```python
from build123d import *

# Parameters (mm, degrees)
SKETCH1_W           = 82
SKETCH1_H           = 38
MAIN_DEPTH          = 3
SKETCH2_W           = 72.5
SKETCH2_H           = 25.5
LCD_CUTOUT_DEPTH    = 46.287967497
SKETCH3_W           = 41
SKETCH3_H           = 4.75
CONNECTOR_CUT_DEPTH = 1.5
SKETCH4_W           = 9.33307462
SKETCH4_H           = 11
CUT_EXTRUDE3_DEPTH  = 46.287967497
SKETCH6_W           = 82
SKETCH6_H           = 38
BOSS_EXTRUDE2_DEPTH = 2
SKETCH7_W           = 80.5
SKETCH7_H           = 36.5
CUT_EXTRUDE6_DEPTH  = 46.287967497
SKETCH8_W           = 41
SKETCH8_H           = 4.75
CUT_EXTRUDE7_DEPTH  = 46.323834789
SKETCH9_W           = 0.75
SKETCH9_H           = 11
BOSS_EXTRUDE3_DEPTH = 3
SKETCH10_W          = 38
SKETCH10_H          = 5
CUT_EXTRUDE8_DEPTH  = 1.2


with BuildPart() as part:
    # Sketch1 → main (new body)
    with BuildSketch(Plane(origin=(0, 0, 0), x_dir=(1, 0, 0), z_dir=(0, 1, 0))):
        Rectangle(SKETCH1_W, SKETCH1_H)
    extrude(amount=MAIN_DEPTH)

    # Sketch2 → LCD cutout (cut, through all)
    with BuildSketch(Plane(origin=(0, 3, 0), x_dir=(1, 0, 0), z_dir=(0, 1, 0))):
        Rectangle(SKETCH2_W, SKETCH2_H)
    extrude(amount=-LCD_CUTOUT_DEPTH, mode=Mode.SUBTRACT)

    # Sketch3 → connector cut (cut)
    with BuildSketch(Plane.XZ):
        with Locations((-14.5, -16.625)):
            Rectangle(SKETCH3_W, SKETCH3_H)
    extrude(amount=-CONNECTOR_CUT_DEPTH, mode=Mode.SUBTRACT)

    # Sketch4 → Cut-Extrude3 (cut, through all)
    with BuildSketch(Plane(origin=(0, 3, 0), x_dir=(1, 0, 0), z_dir=(0, 1, 0))):
        with Locations((36.888390736, 0)):
            Rectangle(SKETCH4_W, SKETCH4_H)
    extrude(amount=-CUT_EXTRUDE3_DEPTH, mode=Mode.SUBTRACT)

    # Sketch6 → Boss-Extrude2 (add)
    with BuildSketch(Plane(origin=(0, 0, 0), x_dir=(1, 0, 0), z_dir=(0, 1, 0))):
        Rectangle(SKETCH6_W, SKETCH6_H)
    extrude(amount=-BOSS_EXTRUDE2_DEPTH)

    # Sketch7 → Cut-Extrude6 (cut, through all)
    with BuildSketch(Plane(origin=(0, 0, 0), x_dir=(1, 0, 0), z_dir=(0, 1, 0))):
        Rectangle(SKETCH7_W, SKETCH7_H)
    extrude(amount=-CUT_EXTRUDE6_DEPTH, mode=Mode.SUBTRACT)

    # Sketch8 → Cut-Extrude7 (cut, through all)
    with BuildSketch(Plane.XZ.offset(-1.5)):
        with Locations((-14.5, -16.625)):
            Rectangle(SKETCH8_W, SKETCH8_H)
    extrude(amount=CUT_EXTRUDE7_DEPTH, mode=Mode.SUBTRACT)

    # Sketch9 → Boss-Extrude3 (add)
    with BuildSketch(Plane(origin=(0, 0, 0), x_dir=(1, 0, 0), z_dir=(0, 1, 0))):
        with Locations((40.625, 0)):
            Rectangle(SKETCH9_W, SKETCH9_H)
    extrude(amount=BOSS_EXTRUDE3_DEPTH)

    # Sketch10 → Cut-Extrude8 (cut)
    with BuildSketch(Plane.ZY.offset(41)):
        with Locations((0, 0.5)):
            Rectangle(SKETCH10_W, SKETCH10_H)
    extrude(amount=-CUT_EXTRUDE8_DEPTH, mode=Mode.SUBTRACT)


solid = part.part
```
Work out the finished part from the listing and answer in its coordinate system (mm). A direction names the side the tool comes from. Give positions to 0.01 mm unless a question says otherwise; leave off trailing zeros. Order: outer loops, then holes, each group sorted by start corner. A loop starts at its lowest first (then second) coordinate and runs counter-clockwise, first axis right, second up. Notation, with made-up numbers: (76.25, -26.75) - (125.25, -26.75) arc R29 ccw to (125.25, 9.25) - close; hole circle Ø1 at (28, 51.5). An arc over 180 degrees is marked (long way). One line per item, written item: value. Start each with the question number.
1. Consider line 1 (Z direction, x = -18, y = 1.4); line 2 (Z direction, x = 34, y = 1.05); line 3 (X direction, y = 0.7, z = 8.5). Determine where each line is inside the solid, lowest interval first.
2. Each of these flat-tipped pins is pushed along its axis until it touches: pin 1 Ø5 at (x, z) = (-19.5, -16.5) entering from -Y; pin 2 Ø0.6 at (x, y) = (-7, -1.5) entering from -Z; pin 3 Ø1.6 at (x, y) = (-6.5, 1) entering from -Z. Where does it stop, or does it pass through?
3. Section A-A, the plane z = -7 is taken. Write down the section's boundary in (x, y).
4. Section C-C, the plane y = -0.85 is taken. Write down the section's boundary in (x, z), then the cut area to 3 significant figures.
5. For a pull along Z with two mould halves and no side action, classify faces 5 (the face through (-15, 1.5, -17)), 6 (the face through (-15, 1, -14.25)), 7 (the face through (-37, -1, -18.25)), 8 (the face through (40.25, 0, 0)) as released by +Z, released by -Z, zero draft, split by the parting line, or undercut.
6. Section B-B, the plane x = 29 is taken. Write down the section's boundary in (y, z).
7. Which of the six approach directions +Z, -Z, +X, -X, +Y, -Y give full straight-line access (tool end or side, diameter ignored) to faces 1 (the face through (9, 1, -19)), 2 (the face through (0, -1, 18.25)), 3 (the face through (-1, 2, 12.75)), 4 (the face through (-35, 1, -17))?
Filled sheet:
1. line 1: -14.25 to -12.75, 12.75 to 19
1. line 2: -19 to -12.75, 12.75 to 19
1. line 3: -39.8 to -36.25, 36.25 to 41
2. pin 1: y = 0
2. pin 2: z = 18.25
2. pin 3: z = -19
3. outline: (-39.8, 0) - (-36.25, 0) - (-36.25, 3) - (-39.8, 3) - close; (36.25, 0) - (40.25, 0) - (40.25, -2) - (41, -2) - (41, 3) - (36.25, 3) - close
4. outline: (-39.8, -19) - (-35, -19) - (-35, -18.25) - (-39.8, -18.25) - close; (-39.8, 18.25) - (40.25, 18.25) - (40.25, -18.25) - (6, -18.25) - (6, -19) - (41, -19) - (41, 19) - (-39.8, 19) - close
4. area: 118 mm²
5. face 5: zero draft
5. face 6: released by -Z
5. face 7: undercut
5. face 8: undercut
6. outline: (-2, -19) - (3, -19) - (3, -12.75) - (0, -12.75) - (0, -18.25) - (-2, -18.25) - close; (-2, 18.25) - (0, 18.25) - (0, 12.75) - (3, 12.75) - (3, 19) - (-2, 19) - close
7. face 1: -Z, +X, -X, +Y, -Y
7. face 2: -X, -Y
7. face 3: +Y, -Y
7. face 4: -Z, -Y
